Job drawing, mm, ordinate dimensions from the low corner. One solid piece. Give positions to 0.01 mm unless a question says otherwise; leave off trailing zeros. Order: outer loops, then holes, each group sorted by start corner. A loop starts at its lowest first (then second) coordinate and runs counter-clockwise, first axis right, second up. Notation, with made-up numbers: (70.25, 56) -> (121.25, 56) arc R17 ccw to (121.25, 88) -> close; hole circle Ø8 at (0, 76). An arc over 180 degrees is marked (long way). Write item = value, one per line. Start each with the question number.
(1) Probe line 1 along Y through (x, z) = (86.5, 2.7) (1 decimal); line 2 along X through (y, z) = (88, 4.4) (1 decimal); line 3 along X through (y, z) = (31.5, 3.1). List the from-to ranges inside material, lowest first. Write a range as from..to.
(2) Saw through at B-B, the plane y = 20.5. List the corners of the cut face in (x, z), then the cut area to 3 significant figures.
(3) Saw through at A-A, the plane x = 79. List the corners of the cut face in (y, z), then the cut area to 3 significant figures.
(4) Saw through at D-D, the plane x = 91.5. List the corners of the cut face in (y, z).
(5) Flat gauge pins, fed straight in: pin 1 (2.5 mm diameter, centred on y = 103, z = 1.5, fed in from -X); pin 2 (1.4 mm diameter, centred on y = 76.5, z = 2, fed in from +X); pin 3 (1 mm diameter, centred on x = 50.5, y = 84.5, fed in from +Z); pin 4 (2.5 mm diameter, centred on x = 88, z = 3.5, fed in from -Y). Where does each tip first touch, or does it go through?
(6) Two-plate mould, pull along Z, no slides. Class the marked faces 1 and 2: pulls with the +Z half, pulls with the -Z half, needs draft (parallel to the pull), parting line crosses it, or undercut.
(7) Saw through at C-C, the plane x = 18. List the corners of the cut face in (y, z) (1 decimal).
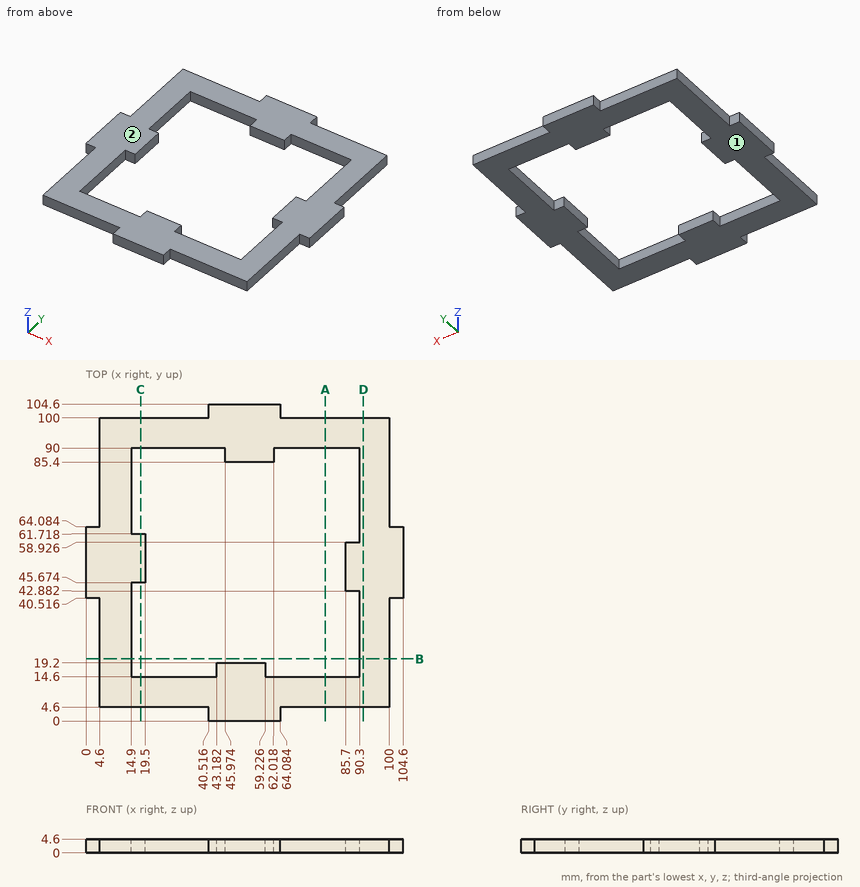
Results list:
q1.line_1 = 4.6..14.6, 42.9..58.9, 90..100
q1.line_2 = 4.6..14.9, 46..62, 90.3..100
q1.line_3 = 4.6..14.9, 90.3..100
q2.outline = (4.6, 0) -> (14.9, 0) -> (14.9, 4.6) -> (4.6, 4.6) -> close; (90.3, 0) -> (100, 0) -> (100, 4.6) -> (90.3, 4.6) -> close
q2.area = 92.0 mm^2
q3.outline = (4.6, 0) -> (14.6, 0) -> (14.6, 4.6) -> (4.6, 4.6) -> close; (90, 0) -> (100, 0) -> (100, 4.6) -> (90, 4.6) -> close
q3.area = 92.0 mm^2
q4.outline = (4.6, 0) -> (100, 0) -> (100, 4.6) -> (4.6, 4.6) -> close
q5.pin_1 = 40.52
q5.pin_2 = 100
q5.pin_3 = through
q5.pin_4 = 4.6
q6.face_1 = pulls with the -Z half
q6.face_2 = pulls with the +Z half
q7.outline = (4.6, 0) -> (14.6, 0) -> (14.6, 4.6) -> (4.6, 4.6) -> close; (45.7, 0) -> (61.7, 0) -> (61.7, 4.6) -> (45.7, 4.6) -> close; (90, 0) -> (100, 0) -> (100, 4.6) -> (90, 4.6) -> close
